Read the model definition and answer for the solid it produces. Units are mm, in the model's axes. A direction names the side the tool comes from. Coordinates: 2 decimals unless noted, no trailing zeros. Loops run counter-clockwise (first coordinate to the right, second up) from the corner with the lowest first, then second, coordinate; pieces in that order, holes last.
Autodesk Inventor part; units mm, degrees
ref_plane "YZ Plane" through (0, 0, 0) normal (1, 0, 0) x (0, 1, 0)
ref_plane "XZ Plane" through (0, 0, 0) normal (0, 1, 0) x (-1, 0, 0)
ref_plane "XY Plane" through (0, 0, 0) normal (0, 0, 1) x (1, 0, 0)
sketch "Sketch1" plane through (0, 0, 0) normal (0, 0, 1) x (1, 0, 0)
  line L0 (-25.5248, 25.2745) -> (-25.2745, -25.5248) construction
  line L1 (-25.2745, -25.5248) -> (25.5248, -25.2745) construction
  line L2 (25.5248, -25.2745) -> (25.2745, 25.5248) construction
  line L3 (25.2745, 25.5248) -> (-25.2745, -25.5248) construction
  line L4 (-25.5248, 25.2745) -> (25.5248, -25.2745) construction
  line L5 (25.2745, 25.5248) -> (48.7045, 49.1868) construction
  line L6 (-25.5248, 25.2745) -> (-49.1868, 48.7045) construction
  line L7 (48.7045, 49.1868) -> (48.7045, 99.9868) construction
  line L8 (-49.1868, 48.7045) -> (-49.1868, 99.5045) construction
  line L9 (-49.1868, 99.5045) -> (-25.6406, 123.0507) construction
  line L10 (48.7045, 99.9868) -> (25.1582, 123.533) construction
  line L11 (-25.6406, 123.0507) -> (-25.6406, 135.7507) construction
  line L12 (25.1582, 123.533) -> (25.1582, 136.233) construction
  line L13 (25.1582, 136.233) -> (19.6449, 167.5007) construction
  line L14 (-25.6406, 135.7507) -> (-20.0422, 167.5007) construction
  line L15 (-20.0422, 167.5007) -> (19.6449, 167.5007) construction
  arc A0 (19.6449, 167.5007) -> (-20.0422, 167.5007) centre (-0.1987, 167.5007) ccw construction
  line L16 (-25.2745, -25.5248) -> (25.5248, -25.2745)
  line L17 (25.5248, -25.2745) -> (25.2745, 25.5248)
  line L18 (48.7045, 49.1868) -> (25.2745, 25.5248)
  line L19 (48.7045, 49.1868) -> (48.7045, 99.9868)
  line L20 (48.7045, 99.9868) -> (25.1582, 123.533)
  line L21 (25.1582, 123.533) -> (25.1582, 136.233)
  line L22 (25.1582, 136.233) -> (19.6449, 167.5007)
  line L23 (-20.0422, 167.5007) -> (-25.6406, 135.7507)
  line L24 (-25.6406, 135.7507) -> (-25.6406, 123.0507)
  line L25 (-25.6406, 123.0507) -> (-49.1868, 99.5045)
  line L26 (-49.1868, 99.5045) -> (-49.1868, 48.7045)
  line L27 (-49.1868, 48.7045) -> (-25.5248, 25.2745)
  line L28 (-25.5248, 25.2745) -> (-25.2745, -25.5248)
  arc A1 (19.6449, 167.5007) -> (-20.0422, 167.5007) centre (-0.1987, 167.5007) ccw
  point P0 (0, 0)
  dimension "d0" = 50.8
  dimension "d1" = 50.8
  dimension "d2" = 33.2994
  dimension "d3" = 33.2994
  dimension "d4" = 135
  dimension "d5" = 135
  dimension "d6" = 50.8
  dimension "d7" = 50.8
  dimension "d8" = 33.2994
  dimension "d9" = 33.2994
  dimension "d10" = 135
  dimension "d11" = 135
  dimension "d12" = 12.7
  dimension "d13" = 12.7
  dimension "d15" = 31.75
  dimension "d16" = 170
  dimension "d17" = 31.75
  dimension "d18" = 170
extrude "Extrusion1" add sketch "Sketch1" along normal blind 6.35
sketch "Sketch2" plane through (0, 0, 0) normal (0, 0, -1) x (-1, 0, 0)
  line L0 (25.2745, -25.5248) -> (-25.5248, -25.2745)
  line L1 (-25.5248, -25.2745) -> (-25.2745, 25.5248)
  arc A0 (20.0422, 167.5007) -> (-19.6449, 167.5007) centre (0.1987, 167.5007) ccw
  line L2 (3.8648, 142.8942) -> (7.531, 136.5442)
  line L3 (7.531, 136.5442) -> (3.8648, 130.1942)
  line L4 (3.8648, 130.1942) -> (-3.4675, 130.1942)
  line L5 (-3.4675, 130.1942) -> (-7.1337, 136.5442)
  line L6 (-7.1337, 136.5442) -> (-3.4675, 142.8942)
  line L7 (-3.4675, 142.8942) -> (3.8648, 142.8942)
  circle A1 centre (0.1987, 136.5442) radius 6.8707
  point P0 (0, 0)
  point P1 (-0.0939, -19.0498)
  point P2 (-0.0939, -6.3498)
  point P3 (-0.0939, 6.3502)
  point P4 (-0.0939, 19.0502)
  point P5 (-0.0939, 31.7502)
  point P6 (12.6061, 31.7502)
  point P7 (-12.7939, 31.7502)
  point P8 (-0.0939, 161.9442)
  point P9 (0.1987, 187.3442)
  point P10 (0.1987, 187.3442)
  point P11 (2.8224, 130.1942)
  point P12 (4.386, 131.097)
  point P13 (7.0098, 135.6415)
  point P14 (7.0098, 137.447)
  point P15 (4.386, 141.9915)
  point P16 (2.8224, 142.8942)
  point P17 (-2.4251, 142.8942)
  point P18 (-3.9887, 141.9915)
  point P19 (-6.6125, 137.447)
  point P20 (-6.6125, 135.6415)
  point P21 (-3.9887, 131.097)
  point P22 (-2.4251, 130.1942)
  dimension "d21" = 6.35
  dimension "d22" = 25.4
  dimension "d23" = 12.7
  dimension "d24" = 12.7
  dimension "d25" = 12.7
  dimension "d26" = 12.7
  dimension "d27" = 12.7
  dimension "d28" = 12.7
  dimension "d29" = 25.4
  dimension "d31" = 25.4
  dimension "d41" = 13.7414
  dimension "d42" = 12.7
hole "Hole1" at (0.0939, -19.0498, 0) at (0.0939, -6.3498, 0) at (0.0939, 6.3502, 0) at (0.0939, 19.0502, 0) at (0.0939, 31.7502, 0) at (-12.6061, 31.7502, 0) at (12.7939, 31.7502, 0) at (0.0939, 161.9442, 0) direction (0, 0, 1) diameter 6.35 end through all
extrude "Extrusion2" cut sketch "Sketch2" against normal blind 6.35 contours L2 A1 L3 L4 L5 L6 L7
equation "\"d3\" = d2"
equation "\"d5\" = d4"
equation "\"d7\" = d6"
equation "\"d11\" = d10"
equation "\"d13\" = d12"
equation "\"d17\" = d15"
equation "\"d18\" = d16"
properties part number "CL1-001" material "Aluminum 6061"
Item 1: Find the intervals of material crossed by line 1 along X through (y, z) = (-7.5, 1.5); line 2 along Y through (x, z) = (-10.5, 4); line 3 along X through (y, z) = (134.5, 5), in increasing order.
Numbers:
line 1: x = -25.36 to -2.87, 3.05 to 25.44
line 2: y = -25.45 to 29.37, 34.13 to 184.46
line 3: x = -25.64 to -6.35, 5.95 to 25.16
Item 2: A cutting plane is placed at C-C on y = 147. Determine the outline of the cut face in (x, z), then the cut area to 3 significant figures.
Numbers:
outline: (-23.66, 0) - (23.26, 0) - (23.26, 6.35) - (-23.66, 6.35) - close
area: 298 mm2
Item 3: Given pin 1 (2.5 mm diameter, centred on x = 1, z = 4.5, fed in from +Y); pin 2 (1 mm diameter, centred on y = 6, z = 3.5, fed in from -X); pin 3 (1 mm diameter, centred on x = 15.5, z = 3, fed in from +Y), each flat-ended and moving along its own axis, determine where each tip first touches the part or whether it passes through.
Numbers:
pin 1: stops at y = 187.34
pin 2: stops at x = -25.43
pin 3: stops at y = 180.26
Item 4: Determine the mould class of faces 3 (the face through (-0.63, 187.34, 3.13)), 4 (the face through (-5.68, 139.75, 3.13)), 5 (the face through (-1, 82, 0)) for opening direction Y: released by +Y, released by -Y, zero draft, split by the parting line, or undercut.
Numbers:
face 3: released by +Y
face 4: undercut
face 5: zero draft
Item 5: A cutting plane is placed at B-B on x = -30. Determine the outline of the cut face in (y, z).
Numbers:
outline: (29.71, 0) - (118.69, 0) - (118.69, 6.35) - (29.71, 6.35) - close
Item 6: A cutting plane is placed at A-A on z = 2.25. Give the number of separate pieces and of enclosed holes in the cut face, then the cut area to 3 significant figures.
Numbers:
separate pieces: 1
enclosed holes: 9
area: 13,400 mm2
Item 7: Which of the six approach directions +Z, -Z, +X, -X, +Y, -Y give full straight-line access (tool end or side, diameter ignored) to faces 1 (the face through (37.096, 111.595, 3.131)), 2 (the face through (5.319, 139.687, 3.131))?
Numbers:
face 1: +Z, -Z, +X, +Y
face 2: +Z, -Z
